```python
from build123d import *

# Parameters (mm, degrees)
PAD004_DEPTH  = 3
PAD003_DEPTH  = 45
FILLET003_R   = 15
FILLET004_R   = 15
BOX006_W      = 192
BOX006_H      = 218
BOX006_DEPTH  = 48
FILLET005_1_R = 15
FILLET005_2_R = 1
PAD007_DEPTH  = 100
PAD005_DEPTH  = 150
CHAMFER_SIZE  = 1.9


with BuildPart() as leftstand:
    # Sketch004 → Pad004 (new body)
    with BuildSketch(Plane.YZ):
        with BuildLine():
            Line((88, 4), (88, 21))
            Line((88, 21), (3, 21))
            Line((3, 21), (3, 0))
            Line((3, 0), (25, 0))
            ThreePointArc((88, 4), (56.461494, 2.606473), (25, 0))
        make_face()
    extrude(amount=PAD004_DEPTH)


with BuildPart() as leftstand_1:
    # Body004 placement: moved
    add(leftstand.part.moved(Location((40, 0, 106))))


with BuildPart() as fusion002:
    # Body005 base: copy of LeftStand
    add(leftstand_1.part)


with BuildPart() as fusion002_1:
    # Body005 placement: moved
    add(fusion002.part.moved(Location((108, 0, 0))))

    # Fusion002: union LeftStand
    add(leftstand_1.part)


with BuildPart() as fillet004:
    # Sketch003 → Pad003 (new body)
    with BuildSketch(Plane.XY):
        with BuildLine():
            Line((18, 0), (168, 0))
            Line((168, 0), (168, 5))
            ThreePointArc((168, 5), (180.727922, 10.272078), (186, 23))
            Line((186, 192), (186, 23))
            ThreePointArc((186, 192), (180.727922, 204.727922), (168, 210))
            Line((18, 210), (168, 210))
            ThreePointArc((18, 210), (5.272078, 204.727922), (0, 192))
            Line((0, 192), (0, 23))
            ThreePointArc((0, 23), (5.272078, 10.272078), (18, 5))
            Line((18, 0), (18, 5))
        make_face()
    extrude(amount=PAD003_DEPTH)


with BuildPart() as fillet004_1:
    # Body003 placement: moved
    add(fillet004.part.moved(Location((3, 3, 82))))

    # Cut001: cut Fusion002
    add(fusion002_1.part, mode=Mode.SUBTRACT)

    # Fillet003
    fillet003_edges = [fillet004_1.edges().sort_by_distance(p)[0] for p in [
        (8.272078, 207.727922, 127),
        (96, 213, 127),
        (3, 110.5, 127),
        (183.727922, 207.727922, 127),
        (189, 110.5, 127),
        (183.727922, 13.272078, 127),
        (95.5, 3, 127),
        (8.272078, 13.272078, 127),
    ]]
    fillet(fillet003_edges, radius=FILLET003_R)

    # Fillet004
    fillet004_edges = [fillet004_1.edges().sort_by_distance(p)[0] for p in [
        (161, 3, 127),
        (30.5, 3, 127),
    ]]
    fillet(fillet004_edges, radius=FILLET004_R)


with BuildPart() as fillet005:
    # Box006 → Box006 (new body)
    with BuildSketch(Plane.XY.offset(82)):
        with Locations((96, 109)):
            Rectangle(BOX006_W, BOX006_H)
    extrude(amount=BOX006_DEPTH)

    # Cut002: cut Fillet004
    add(fillet004_1.part, mode=Mode.SUBTRACT)

    # Fillet005 1
    fillet005_1_edges = [fillet005.edges().sort_by_distance(p)[0] for p in [
        (0, 0, 106),
        (0, 109, 130),
        (0, 218, 106),
        (192, 0, 106),
        (96, 0, 130),
        (96, 218, 130),
        (192, 109, 130),
        (192, 218, 106),
    ]]
    fillet(fillet005_1_edges, radius=FILLET005_1_R)

    # Fillet005 2
    fillet005_2_edges = [fillet005.edges().sort_by_distance(p)[0] for p in [
        (171, 8, 97),
        (21, 8, 97),
        (151, 88, 118.5),
        (151, 14, 106),
        (148, 14, 106),
        (148, 88, 118.5),
        (43, 88, 118.5),
        (43, 14, 106),
        (40, 14, 106),
        (40, 88, 118.5),
        (149.5, 88, 110),
        (41.5, 88, 110),
    ]]
    fillet(fillet005_2_edges, radius=FILLET005_2_R)


with BuildPart() as obj1:
    # Sketch007 → Pad007 (new body)
    with BuildSketch(Plane.YZ):
        Polygon((0, 0), (2, 12), (2, 2), (1, 0), align=None)
    extrude(amount=PAD007_DEPTH)


with BuildPart() as obj1_1:
    # Body008 placement: moved
    add(obj1.part.moved(Location((50, 211, 80))))


with BuildPart() as lid:
    # Sketch005 → Pad005 (new body)
    with BuildSketch(Plane.YZ):
        Polygon((0, 12), (0, 2), (1, 0), (2, 0), align=None)
    extrude(amount=PAD005_DEPTH)


with BuildPart() as lid_1:
    # Body006 placement: moved
    add(lid.part.moved(Location((21, 3, 80))))

    # Fusion003: union Fillet005, obj1
    add(fillet005.part)
    add(obj1_1.part)

    # Chamfer
    chamfer_edges = [lid_1.edges().sort_by_distance(p)[0] for p in [
        (21, 4.5, 80),
        (171, 4.5, 80),
        (50, 211.5, 80),
        (150, 211.5, 80),
    ]]
    chamfer(chamfer_edges, length=CHAMFER_SIZE)


solid = lid_1.part
```
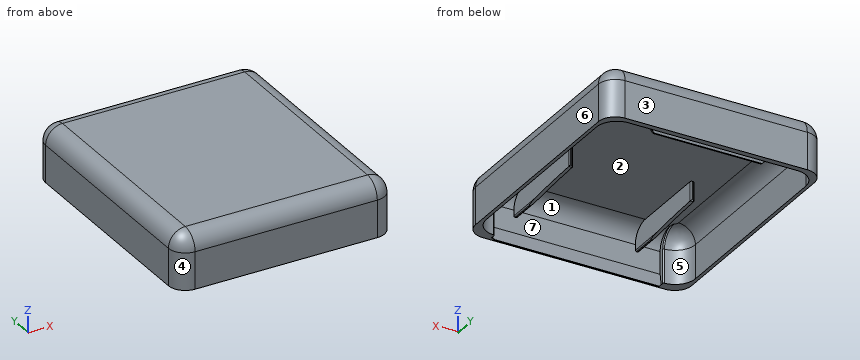
Could you check a few things on this model? Use its own coordinates, in mm. Face numbers are marked on the shaded views. A direction names the side the tool comes from. Give positions to 0.01 mm unless a question says otherwise; leave off trailing zeros. Order: outer loops, then holes, each group sorted by start corner. A loop starts at its lowest first (then second) coordinate and runs counter-clockwise, first axis right, second up.
Q1. Suppose I cut it at D-D, the plane z = 99.5. Write out the boundary of the cut face in (x, y).
Q2. Suppose I cut it at B-B, the plane x = 154. Write out the boundary of the cut face in (y, z).
Q3. If I drill on line 1 along X through (y, z) = (149.5, 93.5); line 2 along Y through (x, z) = (77.5, 111.5); line 3 along Y through (x, z) = (20, 97), over which ranges is the centre line in solid material (lowest first)?
Q4. I'm going to push flat-ended pins straight in: P1, Ø1.9, axis at y = 212.5, z = 86, coming from the -X side; P2, Ø11.5, axis at y = 8, z = 115.5, coming from the +X side; P3, Ø1.1, axis at x = 149.5, y = 10.5, coming from the -Z side. Where does each tip first touch, or does it pass through?
Q5. We'd pull the mould along Y, two halves only. Please class the marked faces 1, 2, 3 and 4: +Y half, -Y half, draft (parallel to the pull), parting line (faces both ways), or undercut.
Q6. Suppose I cut it at A-A, the plane z = 86. Write out the boundary of the cut face in (x, y).
Q7. Suppose I cut it at C-C, the plane y = 177.5. Write out the boundary of the cut face in (x, z), and give its area (3 significant figures).
Q8. For the marked faces 5, 6 and 7, which set-ups out of +Z, -Z, +X, -X, +Y, -Y let a thin tool reach every point of the face, with its end or its side?
Solution:
1. outline: (0, 15) arc R15 ccw to (15, 0) - (177, 0) arc R15 ccw to (192, 15) - (192, 203) arc R15 ccw to (177, 218) - (15, 218) arc R15 ccw to (0, 203) - close; hole (3, 26) arc R18 ccw to (20.05, 8.02) arc R1 cw to (21, 7.03) - (21, 3) - (171, 3) - (171, 7.03) arc R1 cw to (171.95, 8.02) arc R18 ccw to (189, 26) - (189, 195) arc R18 ccw to (171, 213) - (21, 213) arc R18 ccw to (3, 195) - close
2. outline: (0, 82) - (3, 82) - (4, 80) - (5, 80) - (3, 92) - (3, 112) arc R15 cw to (18, 127) - (198, 127) arc R15 cw to (213, 112) - (213, 82) - (218, 82) - (218, 115) arc R15 ccw to (203, 130) - (15, 130) arc R15 ccw to (0, 115) - close
3. line 1: x = 0 to 3, 189 to 192
3. line 2: y = 0 to 3, 213 to 218
3. line 3: y = 0 to 8.03, 212.97 to 218
4. P1: stops at x = 2.68
4. P2: stops at x = 191.95
4. P3: stops at z = 106
5. face 1: undercut
5. face 2: undercut
5. face 3: +Y half
5. face 4: -Y half
6. outline: (0, 15) arc R15 ccw to (15, 0) - (177, 0) arc R15 ccw to (192, 15) - (192, 203) arc R15 ccw to (177, 218) - (15, 218) arc R15 ccw to (0, 203) - close; hole (3, 26) arc R18 ccw to (20.05, 8.02) arc R1 cw to (21, 7.03) - (21, 4) - (171, 4) - (171, 7.03) arc R1 cw to (171.95, 8.02) arc R18 ccw to (189, 26) - (189, 195) arc R18 ccw to (171, 213) - (150, 213) - (150, 212) - (50, 212) - (50, 213) - (21, 213) arc R18 ccw to (3, 195) - close
7. outline: (0, 82) - (3, 82) - (3, 112) arc R15 cw to (18, 127) - (174, 127) arc R15 cw to (189, 112) - (189, 82) - (192, 82) - (192, 115) arc R15 ccw to (177, 130) - (15, 130) arc R15 ccw to (0, 115) - close
7. area: 846 mm2
8. face 5: -Z
8. face 6: +Z, -Z, +X, +Y, -Y
8. face 7: none
